Verification items for this drawing (mm, ordinates from the low corner). A direction names the side the tool comes from. Round coordinates to 2 decimals unless told otherwise and drop trailing zeros. Write each loop counter-clockwise with the first axis right and the second up, starting at its lowest first coordinate (ties: lowest second). Pieces come first, ordered by that corner, then holes. Notation, with made-up numbers: (87.5, 1) -> (115.5, 1) arc R8 ccw to (115.5, 11) -> close; hole circle Ø1 at (37.5, -39.75). An arc over 180 degrees is marked (long way). Put each result on its own line as item: value. Start each with the question number.
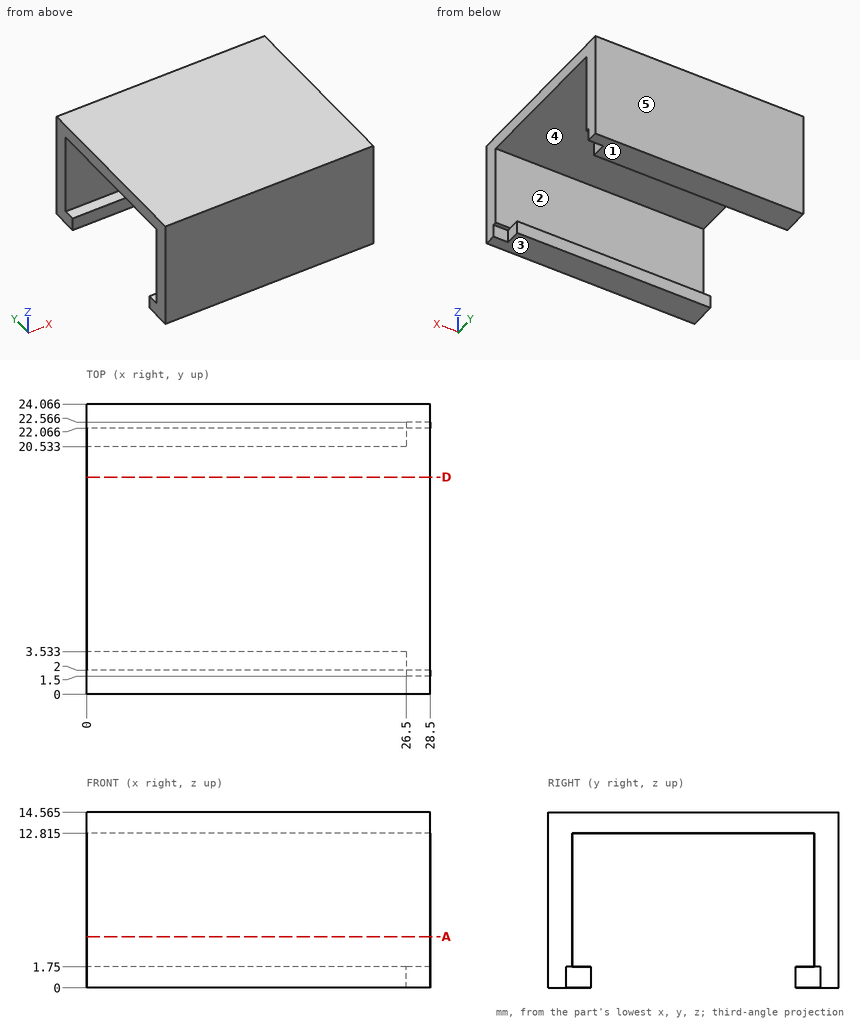
(1) Material ranges on L1, parallel to Y at x = 18.5, z = 3.25; L2, parallel to Z at x = 8.25, y = 14.75 (1 decimal), recorded low to high. Write a range as from..to.
(2) Sectioned sample at D-D (y = 18). Record the cut outline in (x, z) (1 decimal).
(3) Set-up check for the marked faces 1 and 2: record each of +Z, -Z, +X, -X, +Y, -Y from which the full face is reachable in a straight line by a thin tool's end or side.
(4) Mould release check, pull along Y, two halves, no side actions. Record for the marked faces 3, 4 and 5: +Y half, -Y half, draft (parallel to the pull), parting line (faces both ways), or undercut.
(5) Sectioned sample at A-A (z = 4.25). Record the cut outline in (x, y).
(6) Go/stop test with flat-tipped pins: pin 1 Ø10 at (x, y) = (10, 14) entering from -Z (1 decimal); pin 2 Ø0.5 at (y, z) = (22, 1) entering from +X. Record where each tip stops, or that it passes through.
Found:
1. L1: 0..2, 22.07..24.07
1. L2: 12.8..14.6
2. outline: (0, 12.8) -> (28.5, 12.8) -> (28.5, 14.6) -> (0, 14.6) -> close
3. face 1: -Z, +X, -X, +Y, -Y
3. face 2: +X, -X
4. face 3: draft
4. face 4: undercut
4. face 5: +Y half
5. outline: (0, 0) -> (28.5, 0) -> (28.5, 2) -> (0, 2) -> close; (0, 22.07) -> (28.5, 22.07) -> (28.5, 24.07) -> (0, 24.07) -> close
6. pin 1: z = 12.8
6. pin 2: x = 26.5
